```python
from build123d import *

# Parameters (mm, degrees)
DOWELSUPPORT_DEPTH          = 1.905
DOWELSUPPORT_DEPTH_BACK     = 1.27
SKETCH3_R                   = 3.81
SKETCH5_W                   = 6.35
SKETCH5_H                   = 57.15
SLIDERDOWELSUPPORT_DEPTH    = 1.27
SKETCH17_R                  = 1.549999948
SLIDERDOWELCUTOUT_DEPTH     = 26.035
CUT_EXTRUDE2_DEPTH          = 42.370444934
CUT_EXTRUDE2_DEPTH_BACK     = 42.370444934
SKETCH18_W                  = 1.27
SKETCH18_H                  = 38.1
LPATTERN1_COUNT             = 2
LPATTERN1_PITCH             = 25.4
LATERALSUPPORT_DEPTH        = 1.27
SKETCH8_W                   = 6.35
SKETCH8_H                   = 3
TABSUPPORT_DEPTH            = 1.27
STRINGDOWELSUPPORT_START    = -1.27
STRINGDOWELSUPPORT_DEPTH    = 5.715
INTERSUPPORT_DEPTH          = 1.27
SKETCH10_W                  = 6.35
SKETCH10_H                  = 3
TABBASE_DEPTH               = 1.27
SKETCH12_W                  = 6.35
SKETCH12_H                  = 3
TABDRAFT_DEPTH              = 1.73
TABDRAFT_DRAFT              = 5
TABDRAFT_PROFILE_2_DEPTH    = 1.73
TABDRAFT_PROFILE_2_DRAFT    = 5
STRINGDOWELHOLES_DEPTH      = 53.869299342
STRINGDOWELHOLES_DEPTH_BACK = 1.524
SKETCH14_R                  = 1.600000102
PULLEYDOWELHOLE_DEPTH       = 2.921
FILLET1_R                   = 6.35


with BuildPart() as part:
    # Sketch3 → DowelSupport (new, two sides: drawn at the far end of the back side and taken through both)
    with BuildSketch(Plane(origin=(0, 0, 0), x_dir=(0, 0, -1), z_dir=(1, 0, 0)).offset(-DOWELSUPPORT_DEPTH_BACK)):
        with Locations((0, 37.30625)):
            Circle(SKETCH3_R)
    extrude(amount=DOWELSUPPORT_DEPTH + DOWELSUPPORT_DEPTH_BACK)

    # Sketch8 → TabSupport (add, symmetric)
    with BuildSketch(Plane(origin=(0, 0, 0), x_dir=(0, 0, -1), z_dir=(1, 0, 0))):
        with Locations((0, 34.29)):
            Rectangle(SKETCH8_W, SKETCH8_H)
        with Locations((-12.7, 34.29)):
            Rectangle(SKETCH8_W, SKETCH8_H)
    extrude(amount=TABSUPPORT_DEPTH, both=True)


with BuildPart() as body_2:
    # Sketch5 → SliderDowelSupport (new, symmetric)
    with BuildSketch(Plane(origin=(0, 0, 0), x_dir=(0, 0, -1), z_dir=(1, 0, 0))):
        Rectangle(SKETCH5_W, SKETCH5_H)
    extrude(amount=SLIDERDOWELSUPPORT_DEPTH, both=True)

    # Sketch17 → SliderDowelCutout (cut, symmetric)
    with BuildSketch(Plane(origin=(0, 0, 0), x_dir=(1, 0, 0), z_dir=(0, 1, 0))):
        with BuildLine():
            Line((2.032000054, -1.350000094), (2.032000054, 0))
            ThreePointArc((2.032000054, 0), (1.82045896, -0.78168263), (1.243577144, -1.350000094))
            Line((1.243577144, -1.350000094), (2.032000054, -1.350000094))
        make_face()
        with BuildLine():
            Line((2.032000054, 0), (2.032000054, 1.350000094))
            Line((2.032000054, 1.350000094), (1.243577144, 1.350000094))
            ThreePointArc((1.243577144, 1.350000094), (1.82045896, 0.78168263), (2.032000054, 0))
        make_face()
        with Locations((0.482000106, 0)):
            Circle(SKETCH17_R)
    extrude(amount=SLIDERDOWELCUTOUT_DEPTH, both=True, mode=Mode.SUBTRACT)

    # Sketch18 → Cut-Extrude2 (cut, two sides: drawn at the far end of the back side and taken through both)
    with BuildSketch(Plane(origin=(1.27, 0, 0), x_dir=(0, 0, -1), z_dir=(1, 0, 0)).offset(-CUT_EXTRUDE2_DEPTH_BACK)):
        Rectangle(SKETCH18_W, SKETCH18_H)
    extrude(amount=CUT_EXTRUDE2_DEPTH + CUT_EXTRUDE2_DEPTH_BACK, mode=Mode.SUBTRACT)


with BuildPart() as lpattern1_1:
    # LPattern1: pattern copy
    add(body_2.part.moved(Location(Vector(0, 0, 1) * (1 * LPATTERN1_PITCH))))


with BuildPart() as body_4:
    # Sketch6 → LateralSupport (new, symmetric)
    with BuildSketch(Plane(origin=(0, 0, 0), x_dir=(0, 0, -1), z_dir=(1, 0, 0))):
        Polygon((7.392863577, 39.741434671), (5.805363577, 42.491065329), (8.169612929, 43.856065329), (9.523465192, 44.051124423), (10.602965192, 42.181375577), (9.757112929, 41.106434671), align=None)
    extrude(amount=LATERALSUPPORT_DEPTH, both=True)


with BuildPart() as tabsupport_piece_1:
    # of the separate pieces the step leaves, piece 1, a body of its own (tabsupport_pieces)
    add(part.part.solids().sort_by_distance((0, 37.30625, -3.81))[0])


with BuildPart() as tabsupport_piece_2:
    # of the separate pieces the step leaves, piece 2, a body of its own (tabsupport_pieces)
    add(part.part.solids().sort_by_distance((-1.27, 32.79, 9.525))[0])

    # Sketch15 → StringDowelSupport (add)
    with BuildSketch(Plane(origin=(0, 0, 0), x_dir=(0, 0, -1), z_dir=(1, 0, 0)).offset(STRINGDOWELSUPPORT_START)):
        with BuildLine():
            Line((-14.4145, 36.576), (-10.9855, 36.576))
            ThreePointArc((-10.9855, 36.576), (-8.6995, 34.29), (-10.9855, 32.004))
            Line((-10.9855, 32.004), (-14.4145, 32.004))
            ThreePointArc((-14.4145, 32.004), (-16.7005, 34.29), (-14.4145, 36.576))
        make_face()
    extrude(amount=STRINGDOWELSUPPORT_DEPTH)


with BuildPart() as body_2_1:
    add(body_2.part)

    add(lpattern1_1.part)  # InterSupport merges LPattern1_1

    add(body_4.part)  # InterSupport merges body 4

    add(tabsupport_piece_1.part)  # InterSupport merges TabSupport piece 1

    add(tabsupport_piece_2.part)  # InterSupport merges TabSupport piece 2
    # Sketch7 → InterSupport (add, symmetric)
    with BuildSketch(Plane(origin=(0, 0, 0), x_dir=(0, 0, -1), z_dir=(1, 0, 0))):
        Polygon((5.170363577, 43.590917591), (8.027863577, 38.641582409), (1.42875, 34.831582409), (-1.42875, 39.780917591), align=None)
        Polygon((-3.175, 22.225), (-3.175, 28.575), (3.175, 28.575), (3.175, 32.79), (0.923046602, 34.601940251), (-0.923046602, 40.010559749), (-10.9855, 36.576), (-14.4145, 36.576), (-15.109807039, 35.619115541), (-28.575, 28.575), (-22.225, 28.575), (-22.225, 0), (-3.175, 0), align=None)
    extrude(amount=INTERSUPPORT_DEPTH, both=True)

    # Sketch10 → TabBase (add)
    with BuildSketch(Plane.ZY.offset(1.27)):
        with Locations((0, 34.29)):
            Rectangle(SKETCH10_W, SKETCH10_H)
        with Locations((12.7, 34.29)):
            Rectangle(SKETCH10_W, SKETCH10_H)
    extrude(amount=TABBASE_DEPTH)


with BuildPart() as tabdraft_tool:
    # Sketch12 → TabDraft (with draft: the straight prism first)
    with BuildSketch(Plane.ZY.offset(2.54)):
        with Locations((0, 34.29)):
            Rectangle(SKETCH12_W, SKETCH12_H)
    extrude(amount=TABDRAFT_DEPTH)
    # TabDraft: the draft: its side faces are tilted about the plane it starts from
    tabdraft_sides = [tabdraft_tool.faces().sort_by_distance(p)[0] for p in [
        (-3.405, 34.29, 3.175),
        (-3.405, 35.79, 0),
        (-3.405, 34.29, -3.175),
        (-3.405, 32.79, 0),
    ]]
    draft(tabdraft_sides, Plane.ZY.offset(2.54), TABDRAFT_DRAFT)


with BuildPart() as body_2_2:
    add(body_2_1.part)

    # TabDraft: add tabdraft_tool
    add(tabdraft_tool.part)


with BuildPart() as tabdraft_profile_2_tool:
    # Sketch12 → TabDraft profile 2 (with draft: the straight prism first)
    with BuildSketch(Plane.ZY.offset(2.54)):
        with Locations((12.7, 34.29)):
            Rectangle(SKETCH12_W, SKETCH12_H)
    extrude(amount=TABDRAFT_PROFILE_2_DEPTH)
    # TabDraft profile 2: the draft: its side faces are tilted about the plane it starts from
    tabdraft_profile_2_sides = [tabdraft_profile_2_tool.faces().sort_by_distance(p)[0] for p in [
        (-3.405, 34.29, 9.525),
        (-3.405, 32.79, 12.7),
        (-3.405, 34.29, 15.875),
        (-3.405, 35.79, 12.7),
    ]]
    draft(tabdraft_profile_2_sides, Plane.ZY.offset(2.54), TABDRAFT_PROFILE_2_DRAFT)


with BuildPart() as body_2_3:
    add(body_2_2.part)

    # TabDraft profile 2: add tabdraft_profile_2_tool
    add(tabdraft_profile_2_tool.part)

    # Sketch16 → StringDowelHoles (cut, two sides: drawn at the far end of the back side and taken through both)
    with BuildSketch(Plane(origin=(1.905, 0, 0), x_dir=(0, 0, -1), z_dir=(1, 0, 0)).offset(-STRINGDOWELHOLES_DEPTH_BACK)):
        with BuildLine():
            Line((-13.00760401, 33.528), (-12.39239599, 33.528))
            ThreePointArc((-12.39239599, 33.528), (-9.385499898, 34.29), (-12.39239599, 35.052))
            Line((-12.39239599, 35.052), (-13.00760401, 35.052))
            ThreePointArc((-13.00760401, 35.052), (-16.014500102, 34.29), (-13.00760401, 33.528))
        make_face()
    extrude(amount=STRINGDOWELHOLES_DEPTH + STRINGDOWELHOLES_DEPTH_BACK, mode=Mode.SUBTRACT)

    # Sketch14 → PulleyDowelHole (cut)
    with BuildSketch(Plane(origin=(1.905, 0, 0), x_dir=(0, 0, -1), z_dir=(1, 0, 0))):
        with Locations((0, 37.30625)):
            Circle(SKETCH14_R)
    extrude(amount=-PULLEYDOWELHOLE_DEPTH, mode=Mode.SUBTRACT)

    # Mirror1: body 2 across plane


with BuildPart() as body_2_4:
    add(body_2_3.part)
    add(body_2_3.part.mirror(Plane.ZX))

    # Fillet1
    fillet1_edges = [body_2_4.edges().sort_by_distance(p)[0] for p in [
        (0, -28.575, 28.575),
        (0, 28.575, 28.575),
    ]]
    fillet(fillet1_edges, radius=FILLET1_R)


solid = body_2_4.part
```
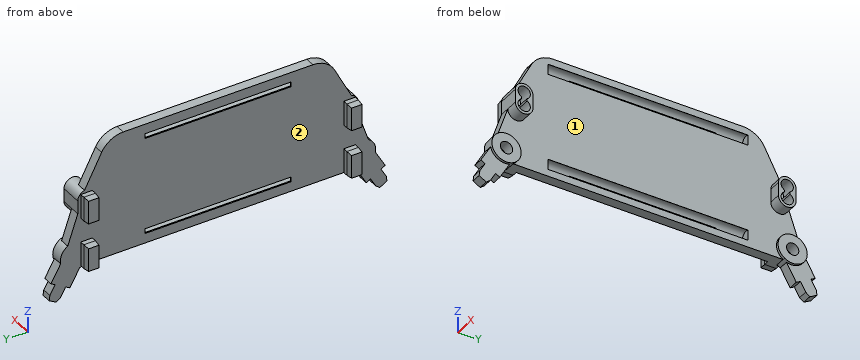
Source: CAD feature listing. Evaluate the final solid. Frame: model axes, mm. Face numbers are marked on the shaded views. Coordinates: 2 decimals unless noted, no trailing zeros. Order: outer loops, then holes, each group sorted by start corner. A loop starts at its lowest first (then second) coordinate and runs counter-clockwise, first axis right, second up. Notation, with made-up numbers: (69, 52) - (119, 52) arc R38 ccw to (119, 90) - close; hole circle Ø10 at (4, -21). An arc over 180 degrees is marked (long way). One line per item, written item: value.
1) Contact query for flat-ended pins moving along their axis: pin 1 (1.4 mm diameter, centred on x = -1.5, z = 11.5, fed in from -Y); pin 2 (1.4 mm diameter, centred on x = -1.5, z = -1, fed in from +Y); pin 3 (4 mm diameter, centred on x = 2, y = -8, fed in from +Z) (3 decimals); pin 4 (2 mm diameter, centred on x = 3, y = -18.5, fed in from -Z). Output: stop coordinate, or through.
Computed values:
pin 1: stops at y = -36.63
pin 2: stops at y = 41.56
pin 3: stops at z = 28.575
pin 4: passes through
2) Ray query, line 1 (Z direction, x = 0, y = -26) (3 decimals); line 2 (Z direction, x = 2.7, y = 34.29); line 3 (Z direction, x = -0.5, y = 19.5) (3 decimals). Return the intervals inside material, ascending. Write a range as [from, to].
Computed values:
line 1: z = [-3.175, -1.473], [1.473, 23.927], [26.873, 28.447]
line 2: z = [8.7, 9.39], [16.01, 16.7]
line 3: z = [-3.175, -1.199], [1.199, 24.201], [26.599, 28.575]
3) Cut plane A-A on y = 3.5. Output: boundary loops of the cut face in (x, z) (3 decimals).
Computed values:
outline: (-1.27, -3.175) - (1.27, -3.175) - (1.27, -1.35) - (1.244, -1.35) arc R1.55 cw to (-0.932, -0.635) - (-1.27, -0.635) - close; (-1.27, 0.635) - (-0.932, 0.635) arc R1.55 cw to (1.244, 1.35) - (1.27, 1.35) - (1.27, 24.05) - (1.244, 24.05) arc R1.55 cw to (-0.932, 24.765) - (-1.27, 24.765) - close; (-1.27, 26.035) - (-0.932, 26.035) arc R1.55 cw to (1.244, 26.75) - (1.27, 26.75) - (1.27, 28.575) - (-1.27, 28.575) - close
4) Cut plane B-B on z = 17.5. Output: boundary loops of the cut face in (x, y).
Computed values:
outline: (-1.27, -34.37) - (1.27, -34.37) - (1.27, 34.37) - (-1.27, 34.37) - close
5) Mould query, pull axis Y, two halves, no side actions, for the marked faces 1 and 2. Classes: released by +Y, released by -Y, zero draft, split by the parting line, or undercut.
Computed values:
face 1: undercut
face 2: undercut
